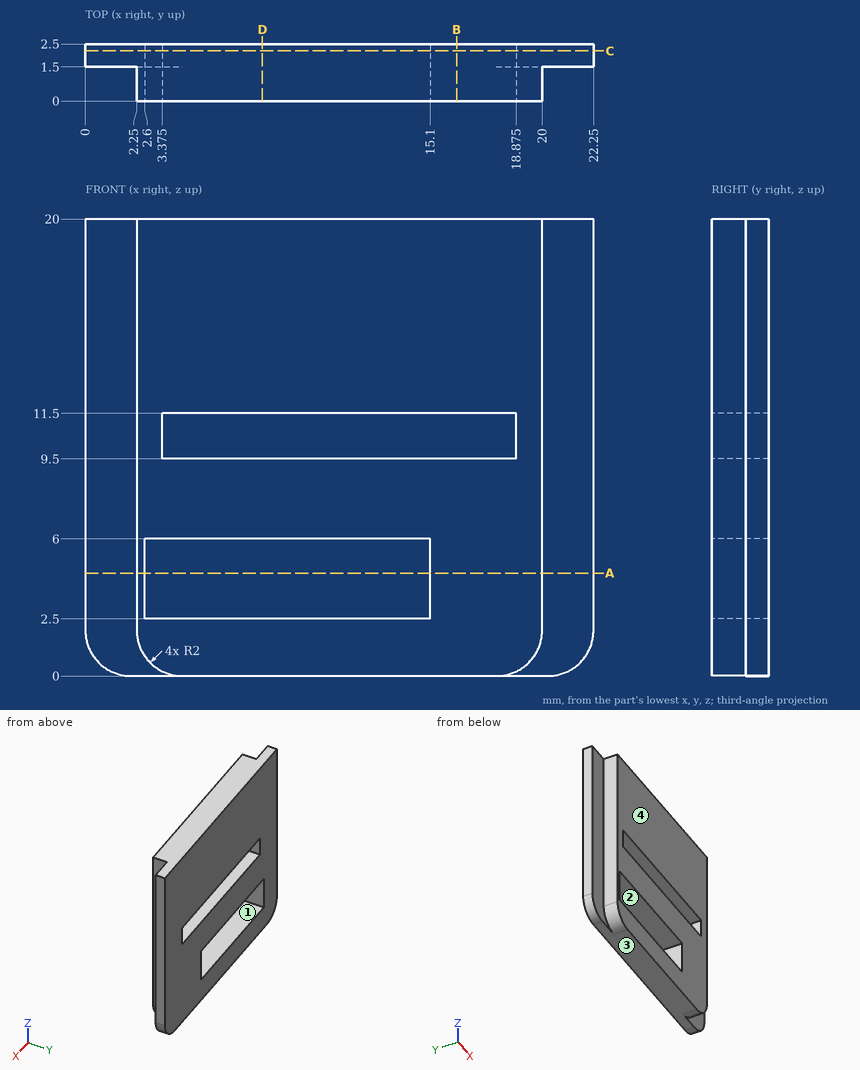
The figure shows three views and two pictorial views of one solid part (mm, origin at its lowest corner). Answer the questions. Round coordinates to 2 decimals unless told otherwise and drop trailing zeros. Order: outer loops, then holes, each group sorted by start corner. A loop starts at its lowest first (then second) coordinate and runs counter-clockwise, first axis right, second up. Notation, with made-up numbers: M -31.75,25.5 L -15.75,25.5 A17 ccw -15.75,35.5 Z; hole C 31.5,48 d10. An arc over 180 degrees is marked long. Answer in a Markdown table with one row per item. Add a question column.
1) The part is cut by section C-C on y = 2.2. Determine the outline of the cut face in (x, z) (3 decimals), plus the area to 3 significant figures.
2) Determine the mould class of the marked faces 1, 2, 3 and 4 for opening direction Z: pulls with the +Z half, pulls with the -Z half, needs draft (parallel to the pull), parting line crosses it, or undercut.
3) Consider line 1 along Z through (x, y) = (12.25, 2.2); line 2 along X through (y, z) = (0.85, 4.25); line 3 along X through (y, z) = (1.25, 10.5) (3 decimals). Determine where each line is inside the solid, lowest interval first. Write a range as from..to.
4) The part is cut by section A-A on z = 4.5. Determine the outline of the cut face in (x, y).
5) Flat-ended cylindrical pins translate along their axes: pin 1 Ø1.3 at (x, z) = (20.5, 7) entering from -Y; pin 2 Ø0.6 at (y, z) = (1, 10.5) entering from -X. Find the tip coordinate at first contact, or state that the pin passes through.
6) The part is cut by section D-D on x = 7.75. Determine the outline of the cut face in (y, z), plus the area to 4 significant figures.
7) The part is cut by section B-B on x = 16.25. Determine the outline of the cut face in (y, z), plus the area to 3 significant figures.
Findings below:
| question | item | result |
|---|---|---|
| 1 | outline | M 0,2 A2 ccw 2,0 L 20.25,0 A2 ccw 22.25,2 L 22.25,20 L 0,20 Z; hole M 2.6,2.5 L 15.1,2.5 L 15.1,6 L 2.6,6 Z; hole M 3.375,9.5 L 18.875,9.5 L 18.875,11.5 L 3.375,11.5 Z |
| 1 | area | 369 mm² |
| 2 | face 1 | undercut |
| 2 | face 2 | undercut |
| 2 | face 3 | pulls with the -Z half |
| 2 | face 4 | needs draft |
| 3 | line 1 | z = 0..2.5, 6..9.5, 11.5..20 |
| 3 | line 2 | x = 2.25..2.6, 15.1..20 |
| 3 | line 3 | x = 2.25..3.375, 18.875..20 |
| 4 | outline | M 0,1.5 L 2.25,1.5 L 2.25,0 L 2.6,0 L 2.6,2.5 L 0,2.5 Z; M 15.1,0 L 20,0 L 20,1.5 L 22.25,1.5 L 22.25,2.5 L 15.1,2.5 Z |
| 5 | pin 1 | stops at y = 0 |
| 5 | pin 2 | stops at x = 2.25 |
| 6 | outline | M 0,0 L 2.5,0 L 2.5,2.5 L 0,2.5 Z; M 0,6 L 2.5,6 L 2.5,9.5 L 0,9.5 Z; M 0,11.5 L 2.5,11.5 L 2.5,20 L 0,20 Z |
| 6 | area | 36.25 mm² |
| 7 | outline | M 0,0 L 2.5,0 L 2.5,9.5 L 0,9.5 Z; M 0,11.5 L 2.5,11.5 L 2.5,20 L 0,20 Z |
| 7 | area | 45.0 mm² |
